from build123d import *

# Parameters (mm, degrees)
BOSS_EXTRUDE1_DEPTH = 2.54


with BuildPart() as part:
    # Sketch1 → Boss-Extrude1 (new body)
    with BuildSketch(Plane(origin=(0, 0, 0), x_dir=(1, 0, 0), z_dir=(0, 1, 0))):
        Polygon((0.6, 11.5), (-20.8, 11.5), (-20.8, -13.5), (32, -13.5), (32, 11.5), (10.6, 11.5), (10.6, 8.5), (0.6, 8.5), align=None)
        with BuildLine():
            Line((11.6, -8.5), (-0.4, -8.5))
            Line((-0.4, -8.5), (-0.4, -4.04977477))
            ThreePointArc((-0.4, -4.04977477), (-15.284741902, 4.449576241), (1.6, 1.5))
            ThreePointArc((1.6, 1.5), (1.352975635, -0.558446724), (0.625930365, -2.5))
            Line((0.625930365, -2.5), (10.574069635, -2.5))
            ThreePointArc((10.574069635, -2.5), (16.241553276, 9.952975635), (27, 1.5))
            ThreePointArc((27, 1.5), (21.249576241, -6.684741902), (11.6, -4.04977477))
            Line((11.6, -4.04977477), (11.6, -8.5))
        make_face(mode=Mode.SUBTRACT)
    extrude(amount=BOSS_EXTRUDE1_DEPTH)


solid = part.part
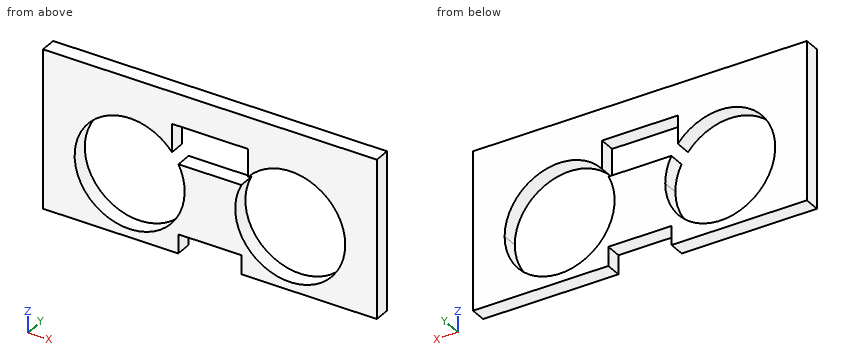
Could you check a few things on this model? Use its own coordinates, in mm. Give positions to 0.01 mm unless a question says otherwise; leave off trailing zeros. Order: outer loops, then holes, each group sorted by start corner. A loop starts at its lowest first (then second) coordinate and runs counter-clockwise, first axis right, second up. Notation, with made-up numbers: M -7.5,22 L 5.5,22 A28 cw 5.5,45 Z; hole C 73.25,16 d4. An arc over 180 degrees is marked long. One line per question, with ' | ' between items.
1. If I drill on line 1 (Z direction, x = -7.1, y = 1.75); line 2 (X direction, y = 1.45, z = -1.5); line 3 (X direction, y = 0.3, z = 0.75), over which ranges is the centre line in solid material (lowest first)?
Results:
line 1: -11.5 to -10.2, 7.2 to 13.5 | line 2: -20.8 to -15.8, 1.6 to 9.6, 27 to 32 | line 3: -20.8 to -15.5, 1.3 to 9.9, 26.7 to 32
2. I want a section at D-D (z = 6.25). List the corners of the cut face in (x, y) for me.
Results:
outline: M -20.8,0 L -11.05,0 L -11.05,2.54 L -20.8,2.54 Z; M -3.15,0 L -0.4,0 L -0.4,2.54 L -3.15,2.54 Z; M 11.6,0 L 14.35,0 L 14.35,2.54 L 11.6,2.54 Z; M 22.25,0 L 32,0 L 32,2.54 L 22.25,2.54 Z
3. I'm going to push a flat-ended pin straight in: pin 1 (1.3 mm diameter, centred on x = 4, y = 1.5, fed in from -Z). Where does the tip first touch, or does it pass through?
Results:
pin 1: z = -8.5
4. I want a section at C-C (z = 3.5). List the corners of the cut face in (x, y) for me.
Results:
outline: M -20.8,0 L -14.22,0 L -14.22,2.54 L -20.8,2.54 Z; M 25.42,0 L 32,0 L 32,2.54 L 25.42,2.54 Z
5. I want a section at B-B (y = 0.9). List the corners of the cut face in (x, z) for me.
Results:
outline: M -20.8,-11.5 L 0.6,-11.5 L 0.6,-8.5 L 10.6,-8.5 L 10.6,-11.5 L 32,-11.5 L 32,13.5 L -20.8,13.5 Z; hole M -0.4,4.05 A8.7 ccw long 0.63,2.5 L 10.57,2.5 A8.7 ccw long 11.6,4.05 L 11.6,8.5 L -0.4,8.5 Z
6. I want a section at A-A (x = 6). List the corners of the cut face in (y, z) for me, and give its area (3 significant figures).
Results:
outline: M 0,-8.5 L 2.54,-8.5 L 2.54,2.5 L 0,2.5 Z; M 0,8.5 L 2.54,8.5 L 2.54,13.5 L 0,13.5 Z | area: 40.6 mm²
